Autodesk Inventor part; units mm, degrees
ref_plane "YZ Plane" through (0, 0, 0) normal (1, 0, 0) x (0, 1, 0)
ref_plane "XZ Plane" through (0, 0, 0) normal (0, 1, 0) x (-1, 0, 0)
ref_plane "XY Plane" through (0, 0, 0) normal (0, 0, 1) x (1, 0, 0)
sketch "Sketch1" plane through (0, 0, 0) normal (0, 0, 1) x (1, 0, 0)
  circle A0 centre (0, 0) radius 4.699
  dimension "d0" = 9.398
extrude "Extrusion1" add sketch "Sketch1" along normal blind 152.4
sketch "Sketch2" plane through (0, 0, 152.4) normal (0, 0, 1) x (1, 0, 0)
  circle A0 centre (0, 0) radius 4.699 construction
  line L0 (-4.699, 0) -> (4.699, 0)
  circle A1 centre (2.54, 0) radius 1.27
  circle A2 centre (-2.54, 0) radius 1.27
  dimension "d3" = 2.54
  dimension "d4" = 2.54
  dimension "d5" = 2.54
  dimension "d6" = 2.54
extrude "Extrusion2" add sketch "Sketch2" along normal blind 190.5
equation "\"d3\" = d4"
properties part number "3618K448"
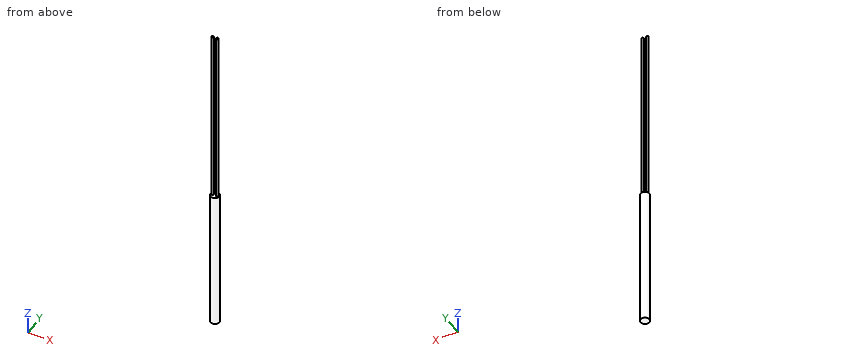
Geometry check sheet. Reference: the model listing, model coordinates, mm. Give positions to 0.01 mm unless a question says otherwise; leave off trailing zeros. Write each loop counter-clockwise with the first axis right and the second up, starting at its lowest first coordinate (ties: lowest second). Pieces come first, ordered by that corner, then holes.
1) Section check A-A, the plane z = 155.5. Record the boundary of the cut face in (x, y).
2) Section check C-C, the plane y = -3. Record the boundary of the cut face in (x, z).
3) Section check B-B, the plane z = 88.5. Record the boundary of the cut face in (x, y), and give its area (3 significant figures).
4) Material ranges on L1, parallel to Z at x = 0.25, y = -2.75; L2, parallel to X at y = -0.5, z = 103.5; L3, parallel to Y at x = 2.5, z = 276, recorded low to high.
5) Gauge pin test, flat ends, axial feed: pin 1 (5 mm diameter, centred on y = -3, z = 281, fed in from -X); pin 2 (2 mm diameter, centred on y = 0.5, z = 225.5, fed in from -X); pin 3 (2 mm diameter, centred on y = 3.5, z = 123, fed in from -X). Record the tip position at first contact, or that the pin passes through.
Computed:
1. outline: circle Ø2.54 at (-2.54, 0); circle Ø2.54 at (2.54, 0)
2. outline: (-3.62, 0) - (3.62, 0) - (3.62, 152.4) - (-3.62, 152.4) - close
3. outline: circle Ø9.4 at (0, 0)
3. area: 69.4 mm2
4. L1: z = 0 to 152.4
4. L2: x = -4.67 to 4.67
4. L3: y = -1.27 to 1.27
5. pin 1: stops at x = -3.71
5. pin 2: stops at x = -3.81
5. pin 3: stops at x = -3.98
